Geometry check sheet. Reference: the model listing, model coordinates, mm. A direction names the side the tool comes from. Give positions to 0.01 mm unless a question says otherwise; leave off trailing zeros. Write each loop counter-clockwise with the first axis right and the second up, starting at its lowest first coordinate (ties: lowest second). Pieces come first, ordered by that corner, then holes. Notation, with made-up numbers: (32, 87.25) -> (46, 87.25) arc R34 cw to (46, 120.25) -> close; hole circle Ø5 at (59, 67). An arc over 180 degrees is marked (long way). One line per item, written item: value.
from build123d import *

# Parameters (mm, degrees)
SKETCH_1_W          = 40
SKETCH_1_H          = 40
SKETCH_1_W_2        = 30.2
SKETCH_1_H_2        = 30.8
EXTRUDE_1_DEPTH     = 2
SKETCH_2_W          = 31.6
SKETCH_2_H          = 33.5
CUT_EXTRUDE_1_DEPTH = 0.5
SKETCH_3_W          = 16
SKETCH_3_H          = 1.2
CUT_EXTRUDE_2_DEPTH = 0.5
FILLET_1_R          = 1
FILLET_2_R          = 2
SKETCH_4_R          = 0.5
EXTRUDE_2_DEPTH     = 1
FILLET_4_R          = 0.5
SKETCH_5_R          = 0.5
CUT_EXTRUDE_3_DEPTH = 1
FILLET_5_R          = 0.5
FILLET_6_R          = 0.5


with BuildPart() as part:
    # 草图1 → 凸台-拉伸1 (new body)
    with BuildSketch(Plane(origin=(0, 0, 0), x_dir=(1, 0, 0), z_dir=(0, 1, 0))):
        Rectangle(SKETCH_1_W, SKETCH_1_H)
        with Locations((0, 1)):
            Rectangle(SKETCH_1_W_2, SKETCH_1_H_2, mode=Mode.SUBTRACT)
    extrude(amount=EXTRUDE_1_DEPTH)

    # 草图2 → 切除-拉伸1 (cut)
    with BuildSketch(Plane.XZ):
        Rectangle(SKETCH_2_W, SKETCH_2_H)
    extrude(amount=-CUT_EXTRUDE_1_DEPTH, mode=Mode.SUBTRACT)

    # 草图3 → 切除-拉伸2 (cut)
    with BuildSketch(Plane.XZ.offset(-0.5)):
        with Locations((0, 15)):
            Rectangle(SKETCH_3_W, SKETCH_3_H)
    extrude(amount=-CUT_EXTRUDE_2_DEPTH, mode=Mode.SUBTRACT)

    # 圆角1
    fillet_1_edges = [part.edges().sort_by_distance(p)[0] for p in [
        (15.1, 2, -1),
        (0, 2, -16.4),
        (-15.1, 2, -1),
        (0, 2, 14.4),
    ]]
    fillet(fillet_1_edges, radius=FILLET_1_R - 0.0001)  # a hair under: the kernel refuses the full size

    # 圆角2
    fillet_2_edges = [part.edges().sort_by_distance(p)[0] for p in [
        (0, 2, -20),
        (20, 2, 0),
        (0, 2, 20),
        (-20, 2, 0),
    ]]
    fillet(fillet_2_edges, radius=FILLET_2_R - 0.0001)  # a hair under: the kernel refuses the full size

    # 草图4 → 凸台-拉伸2 (add)
    with BuildSketch(Plane.XZ):
        with Locations(Location((-19, -19, 0), (0, 0, 270))):
            Circle(SKETCH_4_R)
        with Locations(Location((19, 19, 0), (0, 0, 270))):
            Circle(SKETCH_4_R)
    extrude(amount=EXTRUDE_2_DEPTH)

    # 圆角4
    fillet_4_edges = [part.edges().sort_by_distance(p)[0] for p in [
        (19, -1, 19.5),
    ]]
    fillet(fillet_4_edges, radius=FILLET_4_R)

    # 草图5 → 切除-拉伸3 (cut)
    with BuildSketch(Plane.XZ):
        with Locations(Location((19, -19, 0), (0, 0, 270))):
            Circle(SKETCH_5_R)
        with Locations(Location((-19, 19, 0), (0, 0, 270))):
            Circle(SKETCH_5_R)
    extrude(amount=-CUT_EXTRUDE_3_DEPTH, mode=Mode.SUBTRACT)

    # 圆角5
    fillet_5_edges = [part.edges().sort_by_distance(p)[0] for p in [
        (19, 1, -18.5),
        (-19, 1, 19.5),
    ]]
    fillet(fillet_5_edges, radius=FILLET_5_R)

    # 圆角6
    fillet_6_edges = [part.edges().sort_by_distance(p)[0] for p in [
        (-19, -1, -18.5),
    ]]
    fillet(fillet_6_edges, radius=FILLET_6_R)


solid = part.part
1) Tool access check on faces 1 (the flat face through (0, 2, 16)), 2 (the cylindrical face through (15.401, 1.715, -1.23)), 3 (the flat face through (0, 1, 15)). Record the directions out of +Z, -Z, +X, -X, +Y, -Y that give a thin tool (end or side, any length) a straight path to the whole face; none if there is none.
Verdict:
face 1: +Z, -Z, +X, -X, +Y
face 2: +Y
face 3: -Y
2) Depth check by flat-ended pin: pin 1 Ø1 at (x, z) = (1.5, 15) entering from -Y; pin 2 Ø0.6 at (y, z) = (0.5, -4) entering from +X; pin 3 Ø16 at (x, z) = (7, -2.5) entering from -Y; pin 4 Ø20 at (x, z) = (-10, 9.5) entering from -Y. Enter the tip coordinate at first touch or a pass-through.
Verdict:
pin 1: y = 1
pin 2: x = 19.99
pin 3: through
pin 4: y = 0
3) Mould release check, pull along Z, two halves, no side actions. Record for faces 4 (the cylindrical face through (0.225, 1.715, 14.701)), 5 (the flat face through (-18, 0, 0)), 6 (the cylindrical face through (19.4, -0.2, 18.7)): released by +Z, released by -Z, zero draft, split by the parting line, or undercut.
Verdict:
face 4: undercut
face 5: zero draft
face 6: split by the parting line
4) Scan lines: probe 1 along X at (y, z) = (0.1, -19); probe 2 along X at (y, z) = (0.1, 19); probe 3 along X at (y, z) = (0.2, -17). Record each from-to range of solid material in increasing order.
Verdict:
probe 1: -20 to 18.5, 19.5 to 20
probe 2: -20 to -19.5, -18.5 to 20
probe 3: -19.99 to 19.99
5) Sectioned sample at D-D on y = 1.55. Record the cut outline in (x, z).
Verdict:
outline: (-19.26, -19.26) -> (19.26, -19.26) -> (19.26, 19.26) -> (-19.26, 19.26) -> close; hole (-15.26, -16.56) -> (15.26, -16.56) -> (15.26, 14.56) -> (-15.26, 14.56) -> close
